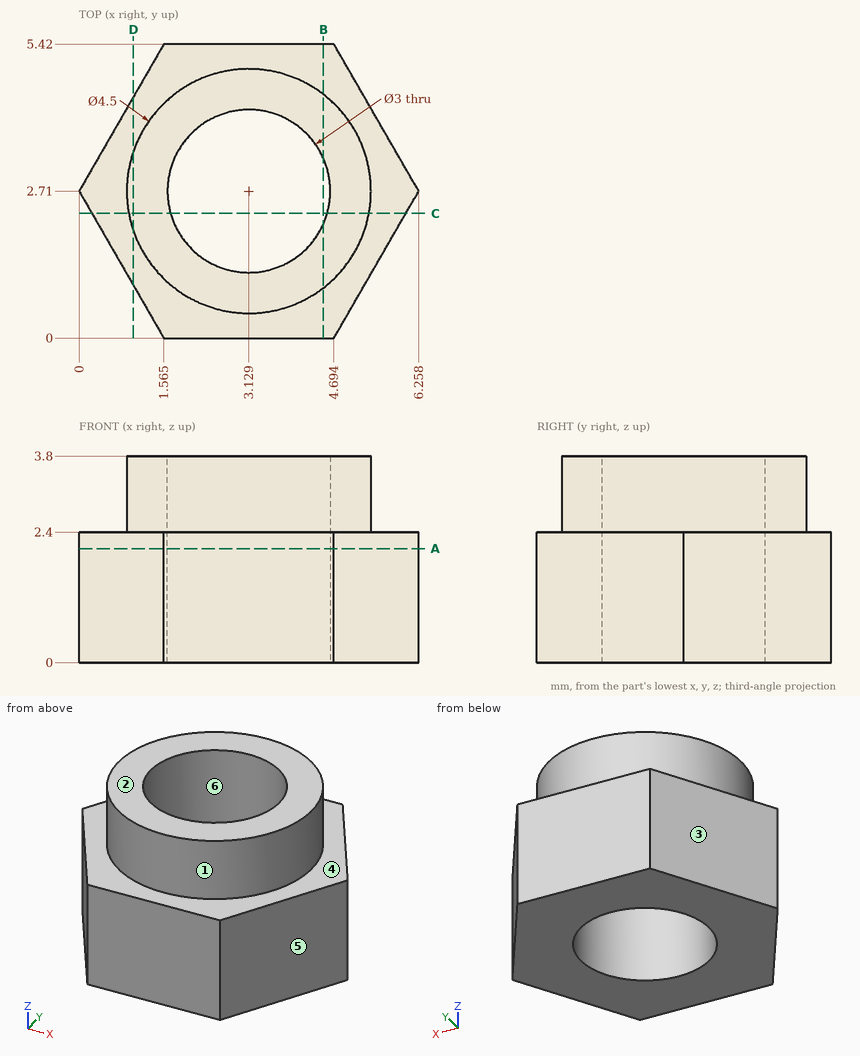
Answer from the drawing. Dimensions are ordinates in mm from the lowest x, y and z of the part. A direction names the side the tool comes from. Give positions to 0.01 mm unless a question says otherwise; leave off trailing zeros. Write each loop counter-clockwise with the first axis right and the second up, starting at its lowest first coordinate (ties: lowest second). Pieces come first, ordered by that corner, then holes. Notation, with made-up numbers: (39, 77) -> (90, 77) arc R35 ccw to (90, 111) -> close; hole circle Ø5 at (62, -38.5). An arc over 180 degrees is marked (long way). Use a Markdown table: item, result.
(1) For the marked faces 1 and 2, determine the directions among +Z, -Z, +X, -X, +Y, -Y from which every point of the face is accessible in a straight line to the end or side of a thin tool.
Return value:
| item | result |
|---|---|
| face 1 | +Z |
| face 2 | +Z, +X, -X, +Y, -Y |
(2) A flat-ended cylindrical pin translates along its axis: P1, Ø2, axis at y = 1.5, z = 0.5, coming from the +X side. Find the tip coordinate at first contact, or state that the pin passes through.
Return value:
| item | result |
|---|---|
| P1 | x = 6.14 |
(3) Section B-B, the plane x = 4.5 is taken. Determine the outline of the cut face in (y, z) (1 decimal).
Return value:
| item | result |
|---|---|
| outline | (0, 0) -> (2.1, 0) -> (2.1, 3.8) -> (0.9, 3.8) -> (0.9, 2.4) -> (0, 2.4) -> close; (3.3, 0) -> (5.4, 0) -> (5.4, 2.4) -> (4.5, 2.4) -> (4.5, 3.8) -> (3.3, 3.8) -> close |
(4) Section A-A, the plane z = 2.1 is taken. Determine the outline of the cut face in (x, y) (1 decimal).
Return value:
| item | result |
|---|---|
| outline | (0, 2.7) -> (1.6, 0) -> (4.7, 0) -> (6.3, 2.7) -> (4.7, 5.4) -> (1.6, 5.4) -> close; hole circle Ø3 at (3.1, 2.7) |
(5) Section C-C, the plane y = 2.3 is taken. Determine the outline of the cut face in (x, z).
Return value:
| item | result |
|---|---|
| outline | (0.24, 0) -> (1.69, 0) -> (1.69, 3.8) -> (0.92, 3.8) -> (0.92, 2.4) -> (0.24, 2.4) -> close; (4.57, 0) -> (6.02, 0) -> (6.02, 2.4) -> (5.34, 2.4) -> (5.34, 3.8) -> (4.57, 3.8) -> close |
(6) Determine the mould class of the marked faces 3, 4, 5 and 6 for opening direction Y: released by +Y, released by -Y, zero draft, split by the parting line, or undercut.
Return value:
| item | result |
|---|---|
| face 3 | released by +Y |
| face 4 | zero draft |
| face 5 | released by -Y |
| face 6 | undercut |
(7) Find the intervals of material crossed by probe 1 along Y at (x, z) = (2.5, 1.65); probe 2 along X at (y, z) = (1.55, 1.85) (1 decimal); probe 3 along X at (y, z) = (1.95, 0.45) (1 decimal), in increasing order. Write a range as from..to.
Return value:
| item | result |
|---|---|
| probe 1 | 0..1.35, 4.07..5.42 |
| probe 2 | 0.7..2.2, 4.1..5.6 |
| probe 3 | 0.4..1.8, 4.4..5.8 |
(8) Section D-D, the plane x = 1 is taken. Determine the outline of the cut face in (y, z).
Return value:
| item | result |
|---|---|
| outline | (0.98, 0) -> (4.44, 0) -> (4.44, 2.4) -> (3.44, 2.4) -> (3.44, 3.8) -> (1.98, 3.8) -> (1.98, 2.4) -> (0.98, 2.4) -> close |
